from build123d import *

# Parameters (mm, degrees)
CUT_EXTRUDE1_REACH  = 23.935
SKETCH2_W           = 2.5
SKETCH2_H           = 1
SKETCH3_W           = 1.5
SKETCH3_H           = 4
BOSS_EXTRUDE1_DEPTH = 5
SKETCH3_3_W         = 2.5
SKETCH3_3_H         = 10
BOSS_EXTRUDE2_DEPTH = 2.5
SKETCH5_R           = 0.5
BOSS_EXTRUDE4_DEPTH = 5


with BuildPart() as part:
    # Sketch1 → Revolve1 (revolve)
    with BuildSketch(Plane.XY, mode=Mode.PRIVATE) as revolve1_sk:
        Polygon((0.030129717, -4.421866179), (1.230129717, -4.421866179), (1.230129717, -0.421866179), (15.030129717, -0.421866179), (15.030129717, 1.078133821), (1.230129717, 1.078133821), (1.030129717, 2.078133821), (1.030129717, 2.578133821), (8.030129717, 2.578133821), (8.030129717, 4.578133821), (5.030129717, 4.578133821), (5.030129717, 5.078133821), (0.030129717, 5.078133821), align=None)
    revolve(revolve1_sk.sketch.rotate(Axis((0.030129717, 5.078133821, 0), (0, -1, 0)), 180), axis=Axis((0.030129717, 5.078133821, 0), (0, -1, 0)))

    # Sketch2 → Cut-Extrude1 (cut, up to next)
    with BuildSketch(Plane.XZ.offset(0.421866179), mode=Mode.PRIVATE) as cut_extrude1_sk1:
        with Locations((-0.492014974, -12.55)):
            Rectangle(SKETCH2_W, SKETCH2_H)
    cut_extrude1_tool1 = extrude(cut_extrude1_sk1.sketch, amount=-CUT_EXTRUDE1_REACH, mode=Mode.PRIVATE) & part.part
    # Sketch2 → Cut-Extrude1 (cut, up to next)
    with BuildSketch(Plane.XZ.offset(0.421866179), mode=Mode.PRIVATE) as cut_extrude1_sk2:
        with Locations((-0.492014974, 12.55)):
            Rectangle(SKETCH2_W, SKETCH2_H)
    cut_extrude1_tool2 = extrude(cut_extrude1_sk2.sketch, amount=-CUT_EXTRUDE1_REACH, mode=Mode.PRIVATE) & part.part
    add(cut_extrude1_tool1.solids().sort_by_distance((-0.492015, -0.421866, -12.55))[0], mode=Mode.SUBTRACT)
    add(cut_extrude1_tool2.solids().sort_by_distance((-0.492015, -0.421866, 12.55))[0], mode=Mode.SUBTRACT)

    # Sketch3 → Boss-Extrude1 (add)
    with BuildSketch(Plane(origin=(0, 1.078133821, 0), x_dir=(1, 0, 0), z_dir=(0, 1, 0))):
        with Locations((-10.25, 0)):
            Rectangle(SKETCH3_W, SKETCH3_H)
    extrude(amount=BOSS_EXTRUDE1_DEPTH)

    # Sketch3<3> → Boss-Extrude2 (add)
    with BuildSketch(Plane(origin=(0, 1.078133821, 0), x_dir=(1, 0, 0), z_dir=(0, 1, 0))):
        with Locations((10.75, 0)):
            Rectangle(SKETCH3_3_W, SKETCH3_3_H)
    extrude(amount=BOSS_EXTRUDE2_DEPTH)

    # Sketch5 → Boss-Extrude4 (add)
    with BuildSketch(Plane(origin=(12, 0, 0), x_dir=(0, 0, -1), z_dir=(1, 0, 0))):
        with Locations(Location((-3.75, 2.328133821, 0), (0, 0, 270))):
            Circle(SKETCH5_R)
        with Locations(Location((-2.25, 2.328133821, 0), (0, 0, 270))):
            Circle(SKETCH5_R)
        with Locations(Location((-0.75, 2.328133821, 0), (0, 0, 270))):
            Circle(SKETCH5_R)
        with Locations(Location((0.75, 2.328133821, 0), (0, 0, 270))):
            Circle(SKETCH5_R)
        with Locations(Location((2.25, 2.328133821, 0), (0, 0, 270))):
            Circle(SKETCH5_R)
        with Locations(Location((3.75, 2.328133821, 0), (0, 0, 270))):
            Circle(SKETCH5_R)
    extrude(amount=BOSS_EXTRUDE4_DEPTH)


solid = part.part
Part model, mm, in its own coordinate system. A direction names the side the tool comes from. Coordinates: 2 decimals unless noted, no trailing zeros. Write each loop counter-clockwise with the first axis right and the second up, starting at its lowest first coordinate (ties: lowest second). Pieces come first, ordered by that corner, then holes. Notation, with made-up numbers: (-17, -18.75) - (-2, -18.75) arc R24 cw to (-2, -5.75) - close; hole circle Ø8 at (-10.5, 50.25). An arc over 180 degrees is marked (long way). Put each result on its own line as item: value.
1. Probe line 1 along Z through (x, y) = (11.5, 3.25); line 2 along Y through (x, z) = (10.5, 7.25); line 3 along Z through (x, y) = (7, 0). List the from-to ranges inside material, lowest first. Write a range as [from, to].
Final values:
line 1: z = [-5, 5]
line 2: y = [-0.42, 1.08]
line 3: z = [-13.28, 13.28]
2. Band-saw the part on D-D (y = -3.5). Write the cut outline in (x, z), then the cut area to 3 significant figures.
Final values:
outline: circle Ø2.4 at (0.03, 0)
area: 4.52 mm²
3. Flat gauge pins, fed straight in: pin 1 Ø0.8 at (x, z) = (11.5, -1.5) entering from +Y; pin 2 Ø2 at (y, z) = (-3, 8) entering from +X; pin 3 Ø4.5 at (y, z) = (4.5, 0.5) entering from +X; pin 4 Ø12 at (x, z) = (8, 10) entering from -Y. Where does each tip first touch, or does it go through?
Final values:
pin 1: stops at y = 3.58
pin 2: passes through
pin 3: stops at x = 17
pin 4: stops at y = -0.42
4. 3-axis set-ups, long thin cutter, end or side, ignore diameter. For faces 4 (the flat face through (-11, 4, 0)), 5 (the flat face through (0.1, 4.578, 5.2)), 6 (the flat face through (-1, 0, -13.05)), 7 (the cylindrical face through (14.465, 2.697, 1.912)): which of +Z, -Z, +X, -X, +Y, -Y reach the whole face in a straight line?
Final values:
face 4: +Z, -Z, -X, +Y
face 5: +Y
face 6: +Y, -Y
face 7: +X
5. Band-saw the part on C-C (z = 6.5). Write the cut outline in (x, y), then the cut area to 3 significant figures.
Final values:
outline: (-13.49, -0.42) - (13.55, -0.42) - (13.55, 1.08) - (-13.49, 1.08) - close; (-4.63, 2.58) - (4.69, 2.58) - (4.69, 4.58) - (-4.63, 4.58) - close
area: 59.2 mm²
6. Two-plate mould, pull along Y, no slides. Class faces 1 (the flat face through (3, -0.422, 0)), 2 (the flat face through (11, 2, 5)), 3 (the flat face through (12, 2, 0)): +Y half, -Y half, draft (parallel to the pull), parting line (faces both ways), or undercut.
Final values:
face 1: -Y half
face 2: draft
face 3: undercut
7. Band-saw the part on A-A (z = -3.75). Write the cut outline in (x, y), then the cut area to 3 significant figures.
Final values:
outline: (-14.49, -0.42) - (14.55, -0.42) - (14.55, 1.08) - (12, 1.08) - (12, 1.83) - (17, 1.83) - (17, 2.83) - (12, 2.83) - (12, 3.58) - (9.5, 3.58) - (9.5, 1.08) - (-14.49, 1.08) - close; (-7.04, 2.58) - (7.1, 2.58) - (7.1, 4.58) - (3.34, 4.58) - (3.34, 5.08) - (-3.28, 5.08) - (-3.28, 4.58) - (-7.04, 4.58) - close
area: 86.4 mm²
8. Band-saw the part on B-B (x = 10). Write the cut outline in (y, z), then the cut area to 3 significant figures.
Final values:
outline: (-0.42, -11.21) - (1.08, -11.21) - (1.08, -5) - (3.58, -5) - (3.58, 5) - (1.08, 5) - (1.08, 11.21) - (-0.42, 11.21) - close
area: 58.6 mm²
